from build123d import *

# Parameters (mm, degrees)
SKETCH_1_W          = 6.6
SKETCH_1_H          = 6.99
SKETCH_1_R          = 1.6
EXTRUDE_1_DEPTH     = 4.88
CUT_EXTRUDE_START   = 4.88
CUT_EXTRUDE_1_DEPTH = 1
CUT_EXTRUDE_2_DEPTH = 0.5
SKETCH_2_R          = 0.23
EXTRUDE_2_DEPTH     = 2.5


with BuildPart() as part:
    # Эскиз1 → Бобышка-Вытянуть1 (new body)
    # profile 1 of 6: a face of its own
    with BuildSketch(Plane(origin=(0, 0, 0), x_dir=(1, 0, 0), z_dir=(0, 1, 0))):
        Rectangle(SKETCH_1_W, SKETCH_1_H)
        Circle(SKETCH_1_R, mode=Mode.SUBTRACT)
    # profile 2 of 6: a face of its own
    with BuildSketch(Plane(origin=(0, 0, 0), x_dir=(1, 0, 0), z_dir=(0, 1, 0))):
        with BuildLine():
            ThreePointArc((0.3, 1.571623365), (0, 1.6), (-0.3, 1.571623365))
            Line((-0.3, 1.571623365), (-0.3, 0.3))
            Line((-0.3, 0.3), (-1.571623365, 0.3))
            ThreePointArc((-1.571623365, 0.3), (-1.6, 0), (-1.571623365, -0.3))
            Line((-1.571623365, -0.3), (-0.3, -0.3))
            Line((-0.3, -0.3), (-0.3, -1.571623365))
            ThreePointArc((-0.3, -1.571623365), (0, -1.6), (0.3, -1.571623365))
            Line((0.3, -1.571623365), (0.3, -0.3))
            Line((0.3, -0.3), (1.571623365, -0.3))
            ThreePointArc((1.571623365, -0.3), (1.592890044, -0.150669534), (1.6, 0))
            ThreePointArc((1.6, 0), (1.592890044, 0.150669534), (1.571623365, 0.3))
            Line((1.571623365, 0.3), (0.3, 0.3))
            Line((0.3, 0.3), (0.3, 1.571623365))
        make_face()
    # profile 3 of 6: a face of its own
    with BuildSketch(Plane(origin=(0, 0, 0), x_dir=(1, 0, 0), z_dir=(0, 1, 0))):
        with BuildLine():
            ThreePointArc((0.3, -1.571623365), (1.13137085, -1.13137085), (1.571623365, -0.3))
            Line((1.571623365, -0.3), (0.3, -0.3))
            Line((0.3, -0.3), (0.3, -1.571623365))
        make_face()
    # profile 4 of 6: a face of its own
    with BuildSketch(Plane(origin=(0, 0, 0), x_dir=(1, 0, 0), z_dir=(0, 1, 0))):
        with BuildLine():
            Line((-0.3, -0.3), (-1.571623365, -0.3))
            ThreePointArc((-1.571623365, -0.3), (-1.13137085, -1.13137085), (-0.3, -1.571623365))
            Line((-0.3, -1.571623365), (-0.3, -0.3))
        make_face()
    # profile 5 of 6: a face of its own
    with BuildSketch(Plane(origin=(0, 0, 0), x_dir=(1, 0, 0), z_dir=(0, 1, 0))):
        with BuildLine():
            Line((-0.3, 0.3), (-0.3, 1.571623365))
            ThreePointArc((-0.3, 1.571623365), (-1.13137085, 1.13137085), (-1.571623365, 0.3))
            Line((-1.571623365, 0.3), (-0.3, 0.3))
        make_face()
    # profile 6 of 6: a face of its own
    with BuildSketch(Plane(origin=(0, 0, 0), x_dir=(1, 0, 0), z_dir=(0, 1, 0))):
        with BuildLine():
            ThreePointArc((1.571623365, 0.3), (1.13137085, 1.13137085), (0.3, 1.571623365))
            Line((0.3, 1.571623365), (0.3, 0.3))
            Line((0.3, 0.3), (1.571623365, 0.3))
        make_face()
    extrude(amount=EXTRUDE_1_DEPTH)

    # Эскиз1<3> → Вырез-Вытянуть1 (cut)
    with BuildSketch(Plane(origin=(0, 0, 0), x_dir=(1, 0, 0), z_dir=(0, 1, 0)).offset(CUT_EXTRUDE_START)):
        with BuildLine():
            ThreePointArc((0.3, 1.571623365), (0, 1.6), (-0.3, 1.571623365))
            Line((-0.3, 1.571623365), (-0.3, 0.3))
            Line((-0.3, 0.3), (-1.571623365, 0.3))
            ThreePointArc((-1.571623365, 0.3), (-1.6, 0), (-1.571623365, -0.3))
            Line((-1.571623365, -0.3), (-0.3, -0.3))
            Line((-0.3, -0.3), (-0.3, -1.571623365))
            ThreePointArc((-0.3, -1.571623365), (0, -1.6), (0.3, -1.571623365))
            Line((0.3, -1.571623365), (0.3, -0.3))
            Line((0.3, -0.3), (1.571623365, -0.3))
            ThreePointArc((1.571623365, -0.3), (1.592890044, -0.150669534), (1.6, 0))
            ThreePointArc((1.6, 0), (1.592890044, 0.150669534), (1.571623365, 0.3))
            Line((1.571623365, 0.3), (0.3, 0.3))
            Line((0.3, 0.3), (0.3, 1.571623365))
        make_face()
    extrude(amount=-CUT_EXTRUDE_1_DEPTH, mode=Mode.SUBTRACT)

    # Эскиз1<4> → Вырез-Вытянуть2 (cut)
    with BuildSketch(Plane(origin=(0, 0, 0), x_dir=(1, 0, 0), z_dir=(0, 1, 0)).offset(CUT_EXTRUDE_START)):
        with BuildLine():
            Line((-0.3, -0.3), (-1.571623365, -0.3))
            ThreePointArc((-1.571623365, -0.3), (-1.13137085, -1.13137085), (-0.3, -1.571623365))
            Line((-0.3, -1.571623365), (-0.3, -0.3))
        make_face()
        with BuildLine():
            Line((-0.3, 0.3), (-0.3, 1.571623365))
            ThreePointArc((-0.3, 1.571623365), (-1.13137085, 1.13137085), (-1.571623365, 0.3))
            Line((-1.571623365, 0.3), (-0.3, 0.3))
        make_face()
        with BuildLine():
            ThreePointArc((1.571623365, 0.3), (1.13137085, 1.13137085), (0.3, 1.571623365))
            Line((0.3, 1.571623365), (0.3, 0.3))
            Line((0.3, 0.3), (1.571623365, 0.3))
        make_face()
        with BuildLine():
            ThreePointArc((0.3, -1.571623365), (1.13137085, -1.13137085), (1.571623365, -0.3))
            Line((1.571623365, -0.3), (0.3, -0.3))
            Line((0.3, -0.3), (0.3, -1.571623365))
        make_face()
    extrude(amount=-CUT_EXTRUDE_2_DEPTH, mode=Mode.SUBTRACT)

    # Эскиз2 → Бобышка-Вытянуть2 (add)
    with BuildSketch(Plane.XZ):
        with Locations(Location((0, 2.575, 0), (0, 0, 90))):
            Circle(SKETCH_2_R)
        with Locations(Location((2.54, 0.035, 0), (0, 0, 90))):
            Circle(SKETCH_2_R)
        with Locations(Location((-2.54, 0.035, 0), (0, 0, 90))):
            Circle(SKETCH_2_R)
    extrude(amount=EXTRUDE_2_DEPTH)


solid = part.part
Geometry check sheet. Reference: the model listing, model coordinates, mm. A direction names the side the tool comes from. Give positions to 0.01 mm unless a question says otherwise; leave off trailing zeros. Loops run counter-clockwise (first coordinate to the right, second up) from the corner with the lowest first, then second, coordinate; pieces in that order, holes last. Notation, with made-up numbers: (16, 84.5) -> (57, 84.5) arc R28 ccw to (57, 104.5) -> close; hole circle Ø1 at (-13.75, 82). An arc over 180 degrees is marked (long way). Answer in a Markdown table with one row per item. Add a question column.
1) Cross-section at B-B on x = 2.54. Record the boundary of the cut face in (y, z) (3 decimals).
2) Set-up check for faces 1 (the face through (-3.3, 2, 0)), 2 (the face through (-1, 4.38, 1)): record each of +Z, -Z, +X, -X, +Y, -Y from which the full face is reachable in a straight line by a thin tool's end or side.
3) Gauge pin test, flat end, axial feed: P1, Ø1.6, axis at x = 0, z = -0.5, coming from the +Y side. Record the tip position at first contact, or that the pin passes through.
4) Draft check along Z on faces 3 (the face through (-1, 4.38, -1)), 4 (the face through (0, 0, 0)), 5 (the face through (0, 2, -3.495)). Enter one of: pulls with the +Z half, pulls with the -Z half, needs draft (parallel to the pull), parting line crosses it, or undercut.
5) Material ranges on probe 1 along X at (y, z) = (4, -1); probe 2 along Z at (x, y) = (1, 4.25) (3 decimals); probe 3 along Y at (x, z) = (-1.5, -1.5), recorded low to high. Write a range as from..to.
6) Cross-section at C-C on x = 1.25. Record the boundary of the cut face in (y, z) (3 decimals).
7) Cross-section at A-A on x = 0. Record the boundary of the cut face in (y, z) (3 decimals).
Outcome:
| question | item | result |
|---|---|---|
| 1 | outline | (-2.5, -0.195) -> (0, -0.195) -> (0, -3.495) -> (4.88, -3.495) -> (4.88, 3.495) -> (0, 3.495) -> (0, 0.265) -> (-2.5, 0.265) -> close |
| 2 | face 1 | +Z, -Z, -X, +Y, -Y |
| 2 | face 2 | +Y |
| 3 | P1 | stops at y = 4.38 |
| 4 | face 3 | undercut |
| 4 | face 4 | needs draft |
| 4 | face 5 | pulls with the -Z half |
| 5 | probe 1 | x = -3.3..-0.3, 0.3..3.3 |
| 5 | probe 2 | z = -3.495..-0.3, 0.3..3.495 |
| 5 | probe 3 | y = 0..4.88 |
| 6 | outline | (0, -3.495) -> (4.88, -3.495) -> (4.88, -0.999) -> (4.38, -0.999) -> (4.38, -0.3) -> (3.88, -0.3) -> (3.88, 0.3) -> (4.38, 0.3) -> (4.38, 0.999) -> (4.88, 0.999) -> (4.88, 3.495) -> (0, 3.495) -> close |
| 7 | outline | (-2.5, 2.345) -> (0, 2.345) -> (0, -3.495) -> (4.88, -3.495) -> (4.88, -1.6) -> (3.88, -1.6) -> (3.88, 1.6) -> (4.88, 1.6) -> (4.88, 3.495) -> (0, 3.495) -> (0, 2.805) -> (-2.5, 2.805) -> close |
